Input: part model. Units: mm. Frame: model coordinates. Face numbers are marked on the shaded views. A direction names the side the tool comes from. Round coordinates to 2 decimals unless told otherwise and drop trailing zeros. Loops run counter-clockwise (first coordinate to the right, second up) from the corner with the lowest first, then second, coordinate; pieces in that order, holes last. Notation, with made-up numbers: M 3,55 L 41,55 A22 cw 41,61 Z; hole C 11,53.5 d1. An arc over 180 degrees is marked long. Put each result on its own line as item: value. Start each with the question number.
1) Section C-C on x = -8. Output: boundary loops of the cut face in (y, z).
2) Reachability of the marked faces 5, 6 and 7 from +Z, -Z, +X, -X, +Y, -Y: full face, straight path, thin tool, end or side. Return the list, or none.
3) Line query: probe 1 along X at (y, z) = (-1, 4.25); probe 2 along Y at (x, z) = (-36.5, 1.5); probe 3 along X at (y, z) = (-0.5, 7). Output: solid intervals per line, ascending.
4) Section D-D on x = 19.5. Output: boundary loops of the cut face in (y, z) (3 decimals), plus the area to 3 significant figures.
5) Draft query along X for the marked faces 1, 2, 3 and 4. Return one class per face: +X half, -X half, draft (parallel to the pull), parting line (faces both ways), or undercut.
6) Pin query (flat end, axial travel): pin 1 (3 mm diameter, centred on y = 0.5, z = 6.5, fed in from +X); pin 2 (5 mm diameter, centred on x = -37.5, z = 3.5, fed in from +Y); pin 3 (1.5 mm diameter, centred on y = 38, z = 4, fed in from -X). Return the tip coordinate at first contact, or that it passes through.
7) Section B-B on z = 6.5. Output: boundary loops of the cut face in (x, y).
8) Section A-A on y = 0. Output: boundary loops of the cut face in (x, z).
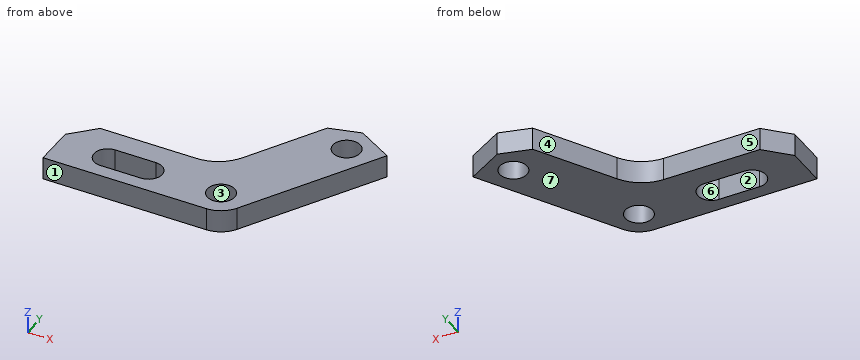
from build123d import *

# Parameters (mm, degrees)
CROQUIS1_R              = 6
SALIENTE_EXTRUIR1_DEPTH = 10


with BuildPart() as part:
    # Croquis1 → Saliente-Extruir1 (new body)
    with BuildSketch(Plane.XY):
        with BuildLine():
            Line((-62, 16), (-19.629909152, 16))
            ThreePointArc((-19.629909152, 16), (-10.629909152, 18.411542732), (-4.041451884, 25))
            Line((-4.041451884, 25), (15.143593539, 58.229473419))
            Line((15.143593539, 58.229473419), (28.803847577, 61.889727457))
            Line((28.803847577, 61.889727457), (44.392304845, 52.889727457))
            Line((44.392304845, 52.889727457), (10.392304845, -6))
            ThreePointArc((10.392304845, -6), (6, -10.392304845), (0, -12))
            Line((0, -12), (-72, -12))
            Line((-72, -12), (-72, 6))
            Line((-72, 6), (-62, 16))
        make_face()
        Circle(CROQUIS1_R, mode=Mode.SUBTRACT)
        with Locations((28.5, 49.363448016)):
            Circle(CROQUIS1_R, mode=Mode.SUBTRACT)
        with BuildLine():
            Line((-32, -6), (-50, -6))
            ThreePointArc((-50, -6), (-56, 0), (-50, 6))
            Line((-50, 6), (-32, 6))
            ThreePointArc((-32, 6), (-26, 0), (-32, -6))
        make_face(mode=Mode.SUBTRACT)
    extrude(amount=SALIENTE_EXTRUIR1_DEPTH)


solid = part.part
Geometry results:
1. outline: M -12,0 L 20.26,0 L 20.26,10 L -12,10 Z
2. face 5: +Z, -Z, -X, +Y
2. face 6: +Z, -Z
2. face 7: -Z, +X, -X, +Y, -Y
3. probe 1: x = -72 to -55.92, -26.08 to -5.92, 5.92 to 13.28
3. probe 2: y = -12 to -6, 6 to 16
3. probe 3: x = -72 to -55.98, -26.02 to -5.98, 5.98 to 13.57
4. outline: M 9.775,0 L 59.397,0 L 59.397,10 L 9.775,10 Z
4. area: 496 mm²
5. face 1: draft
5. face 2: undercut
5. face 3: undercut
5. face 4: -X half
6. pin 1: stops at x = 15.01
6. pin 2: stops at y = 16
6. pin 3: stops at x = 3.03
7. outline: M -72,-12 L 0,-12 A12 ccw 10.39,-6 L 44.39,52.89 L 28.8,61.89 L 15.14,58.23 L -4.04,25 A18 cw -19.63,16 L -62,16 L -72,6 Z; hole M -50,-6 L -32,-6 A6 ccw -32,6 L -50,6 A6 ccw Z; hole C 0,0 d12; hole C 28.5,49.36 d12
8. outline: M -72,0 L -56,0 L -56,10 L -72,10 Z; M -26,0 L -6,0 L -6,10 L -26,10 Z; M 6,0 L 13.86,0 L 13.86,10 L 6,10 Z
